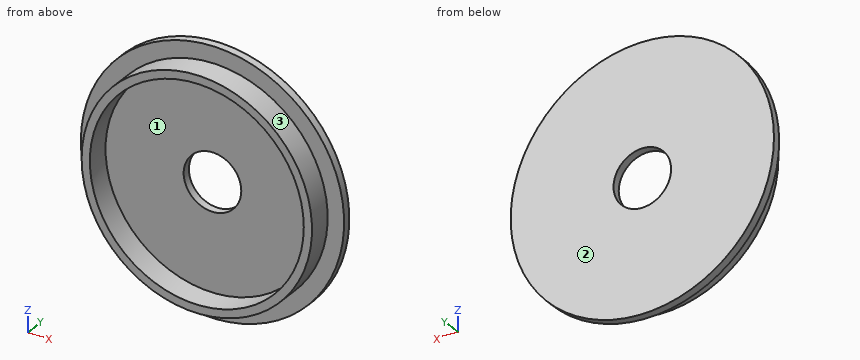
```python
from build123d import *

# Parameters (mm, degrees)
SKETCH2_R          = 41.275
CUT_EXTRUDE1_DEPTH = 9.525
SKETCH3_R          = 11.1125
CUT_EXTRUDE2_DEPTH = 13.7


with BuildPart() as part:
    # Sketch1 → Revolve1 (revolve)
    with BuildSketch(Plane.XY):
        Polygon((0, 0), (-50.8, 0), (-50.8, -3.175), (-44.45, -3.175), (-44.45, -12.7), (0, -12.7), align=None)
    revolve(axis=Axis((0, -12.7, 0), (0, 1, 0)))

    # Sketch2 → Cut-Extrude1 (cut)
    with BuildSketch(Plane.XZ.offset(12.7)):
        Circle(SKETCH2_R)
    extrude(amount=-CUT_EXTRUDE1_DEPTH, mode=Mode.SUBTRACT)

    # Sketch3 → Cut-Extrude2 (cut, through all)
    with BuildSketch(Plane(origin=(0, 0, 0), x_dir=(1, 0, 0), z_dir=(0, 1, 0))):
        Circle(SKETCH3_R)
    extrude(amount=-CUT_EXTRUDE2_DEPTH, mode=Mode.SUBTRACT)


solid = part.part
```
Work out the finished part from the listing and answer in its coordinate system (mm). Face numbers are marked on the shaded views. Give positions to 0.01 mm unless a question says otherwise; leave off trailing zeros. Loops run counter-clockwise (first coordinate to the right, second up) from the corner with the lowest first, then second, coordinate; pieces in that order, holes last. Notation, with made-up numbers: (41.25, 15) -> (95.25, 15) arc R14 ccw to (95.25, 38) -> close; hole circle Ø8 at (-30.5, -14.75). An arc over 180 degrees is marked (long way). One line per question, with ' | ' between items. Start each with the question number.
1) Section D-D, the plane x = 31.5 is taken. Determine the outline of the cut face in (y, z) (3 decimals), then the cut area to 3 significant figures.
2) Section C-C, the plane z = -34 is taken. Determine the outline of the cut face in (x, y) (3 decimals).
3) Determine the mould class of the marked faces 1, 2 and 3 for opening direction Z: +Z half, -Z half, draft (parallel to the pull), parting line (faces both ways), or undercut.
4) Each of these flat-tipped pins is pushed along its axis until it touches: pin 1 (5 mm diameter, centred on x = 4.5, y = -4, fed in from +Z); pin 2 (1 mm diameter, centred on x = 12.5, z = 30, fed in from -Y) (3 decimals); pin 3 (3 mm diameter, centred on y = -6, z = -23, fed in from +X). Where does it stop, or does it pass through?
5) Straight lines are drawn through the part: L1, parallel to X at y = -9.75, z = -1; L2, parallel to Z at x = 0, y = -1.45; L3, parallel to Z at x = 0, y = -7.75 (3 decimals). For each, find the intervals that lie inside material, in ascending order.
Resolved:
1) outline: (-12.7, -31.362) -> (-3.175, -31.362) -> (-3.175, -39.855) -> (0, -39.855) -> (0, 39.855) -> (-3.175, 39.855) -> (-3.175, 31.362) -> (-12.7, 31.362) -> (-12.7, 26.672) -> (-3.175, 26.672) -> (-3.175, -26.672) -> (-12.7, -26.672) -> close | area: 342 mm2
2) outline: (-37.744, -3.175) -> (-28.632, -3.175) -> (-28.632, -12.7) -> (-23.401, -12.7) -> (-23.401, -3.175) -> (23.401, -3.175) -> (23.401, -12.7) -> (28.632, -12.7) -> (28.632, -3.175) -> (37.744, -3.175) -> (37.744, 0) -> (-37.744, 0) -> close
3) face 1: undercut | face 2: draft | face 3: parting line
4) pin 1: z = 50.75 | pin 2: y = -3.175 | pin 3: x = 38.9
5) L1: -44.44 to -41.26, 41.26 to 44.44 | L2: -50.8 to -11.11, 11.11 to 50.8 | L3: -44.45 to -41.275, 41.275 to 44.45
